```python
from build123d import *

# Parameters (mm, degrees)
SKETCH1_R               = 2.5
BOSS_EXTRUDE1_DEPTH     = 26
SKETCH2_R               = 1.25
CUT_EXTRUDE1_DEPTH      = 3.5
CUT_EXTRUDE1_DEPTH_BACK = 3.5


with BuildPart() as part:
    # Sketch1 → Boss-Extrude1 (new body)
    with BuildSketch(Plane.XY):
        with Locations((0.77230809, 0)):
            Circle(SKETCH1_R)
    extrude(amount=BOSS_EXTRUDE1_DEPTH)

    # Sketch2 → Cut-Extrude1 (cut, two sides)
    with BuildSketch(Plane(origin=(0, 0, 0), x_dir=(1, 0, 0), z_dir=(0, 1, 0))) as cut_extrude1_sk:
        with Locations((0.77230809, -3)):
            Circle(SKETCH2_R)
        with Locations((0.77230809, -23)):
            Circle(SKETCH2_R)
    extrude(amount=CUT_EXTRUDE1_DEPTH, mode=Mode.SUBTRACT)
    extrude(cut_extrude1_sk.sketch, amount=-CUT_EXTRUDE1_DEPTH_BACK, mode=Mode.SUBTRACT)


solid = part.part
```
Geometry check sheet. Reference: the model listing, model coordinates, mm. Coordinates: 2 decimals unless noted, no trailing zeros. Loops run counter-clockwise (first coordinate to the right, second up) from the corner with the lowest first, then second, coordinate; pieces in that order, holes last.
Item 1: Release check for a two-part mould opening along Z. For faces 1 (the face through (1, 0, 26)), 2 (the face through (1, 0, 0)) record: released by +Z, released by -Z, zero draft, split by the parting line, or undercut.
Item 2: Sectioned sample at A-A, the plane x = 0.55. Record the boundary of the cut face in (y, z), then the cut area to 3 significant figures.
Item 3: Sectioned sample at B-B, the plane z = 3. Record the boundary of the cut face in (x, y), then the cut area to 3 significant figures.
Item 4: Thickness scan on line 1 (Z direction, x = 1.8, y = 1.1); line 2 (Z direction, x = 0.3, y = -2.1); line 3 (X direction, y = 1.8, z = 23). Record the ranges inside material, lowest first.
Item 5: Sectioned sample at D-D, the plane x = 1.8. Record the boundary of the cut face in (y, z), then the cut area to 3 significant figures.
Item 6: Sectioned sample at C-C, the plane y = -1.9. Record the boundary of the cut face in (x, z), then the cut area to 3 significant figures.
Item 7: Go/stop test with flat-tipped pins: pin 1 Ø1 at (x, z) = (-0.5, 15) entering from -Y; pin 2 Ø2 at (x, z) = (2, 19) entering from +Y. Record where each tip stops, or that it passes through.
Check result:
1. face 1: released by +Z
1. face 2: released by -Z
2. outline: (-2.49, 0) - (2.49, 0) - (2.49, 1.77) - (-2.49, 1.77) - close; (-2.49, 4.23) - (2.49, 4.23) - (2.49, 21.77) - (-2.49, 21.77) - close; (-2.49, 24.23) - (2.49, 24.23) - (2.49, 26) - (-2.49, 26) - close
2. area: 105 mm2
3. outline: (-0.48, -2.17) - (-0.48, 2.17) arc R2.5 ccw to start; (2.02, -2.17) arc R2.5 ccw to (2.02, 2.17) - close
3. area: 7.68 mm2
4. line 1: z = 0 to 2.29, 3.71 to 22.29, 23.71 to 26
4. line 2: z = 0 to 1.84, 4.16 to 21.84, 24.16 to 26
4. line 3: x = -0.96 to -0.48, 2.02 to 2.51
5. outline: (-2.28, 0) - (2.28, 0) - (2.28, 2.29) - (-2.28, 2.29) - close; (-2.28, 3.71) - (2.28, 3.71) - (2.28, 22.29) - (-2.28, 22.29) - close; (-2.28, 23.71) - (2.28, 23.71) - (2.28, 26) - (-2.28, 26) - close
5. area: 106 mm2
6. outline: (-0.85, 0) - (2.4, 0) - (2.4, 26) - (-0.85, 26) - close; hole circle Ø2.5 at (0.77, 3); hole circle Ø2.5 at (0.77, 23)
6. area: 74.7 mm2
7. pin 1: stops at y = -2.38
7. pin 2: stops at y = 2.49
